For this review, take the finished solid that the model builds, in its own axes (mm). Give positions to 0.01 mm unless a question says otherwise; leave off trailing zeros. Order: outer loops, then holes, each group sorted by start corner. A loop starts at its lowest first (then second) coordinate and runs counter-clockwise, first axis right, second up. Notation, with made-up numbers: (-38, 62) - (-22, 62) arc R11 cw to (-22, 76) - close; hole circle Ø4 at (-23.75, 40.25). An arc over 180 degrees is marked (long way). One line per item, written item: value.
```python
from build123d import *

# Parameters (mm, degrees)
BOSS_EXTRUDE1_DEPTH = 5.461
BOSS_EXTRUDE2_DEPTH = 5.461
SKETCH3_W           = 5.461
SKETCH3_H           = 25.4
SKETCH3_W_2         = 19.05
SKETCH3_H_2         = 5.461
CUT_EXTRUDE1_DEPTH  = 6.461
SKETCH4_W           = 25.4
SKETCH4_H           = 10.8204
CUT_EXTRUDE2_DEPTH  = 6.461


with BuildPart() as part:
    # Sketch1 → Boss-Extrude1 (new body)
    with BuildSketch(Plane(origin=(0, 0, 0), x_dir=(1, 0, 0), z_dir=(0, 1, 0))):
        Polygon((-42.3, 45.461), (-99.45, 35.936), (-99.45, -45.979), (60.57, -45.979), (60.57, 45.461), align=None)
        with BuildLine():
            ThreePointArc((-55, 32.5), (-52.803300859, 37.803300859), (-47.5, 40))
            Line((-47.5, 40), (47.5, 40))
            ThreePointArc((47.5, 40), (52.803300859, 37.803300859), (55, 32.5))
            Line((55, 32.5), (55, -32.5))
            ThreePointArc((55, -32.5), (52.803300859, -37.803300859), (47.5, -40))
            Line((47.5, -40), (-47.5, -40))
            ThreePointArc((-47.5, -40), (-52.803300859, -37.803300859), (-55, -32.5))
            Line((-55, -32.5), (-55, 32.5))
        make_face(mode=Mode.SUBTRACT)
    extrude(amount=BOSS_EXTRUDE1_DEPTH)

    # Sketch2 → Boss-Extrude2 (add)
    with BuildSketch(Plane(origin=(0, 5.461, 0), x_dir=(1, 0, 0), z_dir=(0, 1, 0))):
        with BuildLine():
            Line((-47.5, -40), (47.5, -40))
            ThreePointArc((47.5, -40), (52.803300859, -37.803300859), (55, -32.5))
            Line((55, -32.5), (55, 32.5))
            ThreePointArc((55, 32.5), (52.803300859, 37.803300859), (47.5, 40))
            Line((47.5, 40), (-47.5, 40))
            ThreePointArc((-47.5, 40), (-52.803300859, 37.803300859), (-55, 32.5))
            Line((-55, 32.5), (-55, -32.5))
            ThreePointArc((-55, -32.5), (-52.803300859, -37.803300859), (-47.5, -40))
        make_face()
    extrude(amount=-BOSS_EXTRUDE2_DEPTH)

    # Sketch3 → Cut-Extrude1 (cut, through all)
    with BuildSketch(Plane.XZ):
        Polygon((-70.637433485, -40.738094419), (-89.428237734, -37.606293711), (-88.530454864, -32.219596493), (-69.739650615, -35.351397201), align=None)
        with Locations((-96.7195, 5.0215)):
            Rectangle(SKETCH3_W, SKETCH3_H)
        with Locations((-77.225, 43.2485)):
            Rectangle(SKETCH3_W_2, SKETCH3_H_2)
    extrude(amount=-CUT_EXTRUDE1_DEPTH, mode=Mode.SUBTRACT)

    # Sketch4 → Cut-Extrude2 (cut, through all)
    with BuildSketch(Plane(origin=(0, 5.461, 0), x_dir=(1, 0, 0), z_dir=(0, 1, 0))):
        with Locations((-6.35, -20.6375)):
            Rectangle(SKETCH4_W, SKETCH4_H)
        with Locations((-6.35, 20.6375)):
            Rectangle(SKETCH4_W, SKETCH4_H)
    extrude(amount=-CUT_EXTRUDE2_DEPTH, mode=Mode.SUBTRACT)


solid = part.part
```
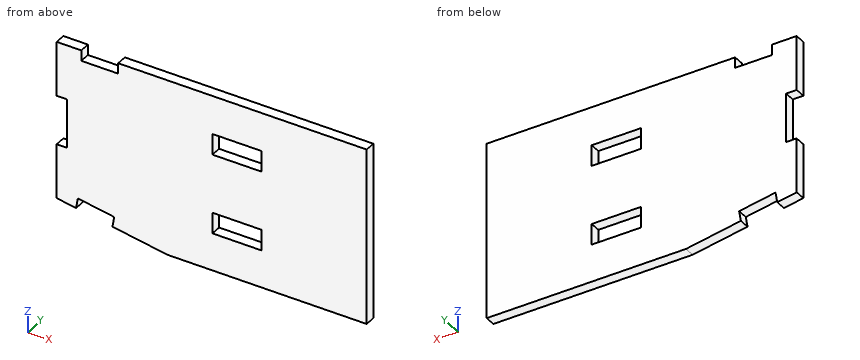
(1) Take a section at B-B (y = 2.15). Write out the cut boundary in (x, z), then the cut area to 3 significant figures.
Answers below:
outline: (-99.45, -35.94) - (-89.43, -37.61) - (-88.53, -32.22) - (-69.74, -35.35) - (-70.64, -40.74) - (-42.3, -45.46) - (60.57, -45.46) - (60.57, 45.98) - (-67.7, 45.98) - (-67.7, 40.52) - (-86.75, 40.52) - (-86.75, 45.98) - (-99.45, 45.98) - (-99.45, 17.72) - (-93.99, 17.72) - (-93.99, -7.68) - (-99.45, -7.68) - close; hole (-19.05, -26.05) - (6.35, -26.05) - (6.35, -15.23) - (-19.05, -15.23) - close; hole (-19.05, 15.23) - (6.35, 15.23) - (6.35, 26.05) - (-19.05, 26.05) - close
area: 13,500 mm^2
(2) For P1, Ø2.5, axis at x = -95.5, y = 3, coming from the -Z side, flat-tipped, find the tip position at first contact; note if it passes through.
Answers below:
P1: stops at z = -36.8
(3) Take a section at D-D (x = -64). Write out the cut boundary in (y, z).
Answers below:
outline: (0, -41.84) - (5.46, -41.84) - (5.46, 45.98) - (0, 45.98) - close
(4) Wall thickness on line 1 (Z direction, x = -3, y = 3.45); line 2 (X direction, y = 2.4, z = -19); line 3 (X direction, y = 4.7, z = 10): over which ranges is each line inside the solid? List them lowest first. Write a range as from..to.
Answers below:
line 1: z = -45.46..-26.05, -15.23..15.23, 26.05..45.98
line 2: x = -99.45..-19.05, 6.35..60.57
line 3: x = -93.99..60.57
(5) Take a section at C-C (z = -6). Write out the cut boundary in (x, y), then the cut area to 3 significant figures.
Answers below:
outline: (-93.99, 0) - (60.57, 0) - (60.57, 5.46) - (-93.99, 5.46) - close
area: 844 mm^2
(6) Take a section at A-A (x = -9.5). Write out the cut boundary in (y, z), then the cut area to 3 significant figures.
Answers below:
outline: (0, -45.46) - (5.46, -45.46) - (5.46, -26.05) - (0, -26.05) - close; (0, -15.23) - (5.46, -15.23) - (5.46, 15.23) - (0, 15.23) - close; (0, 26.05) - (5.46, 26.05) - (5.46, 45.98) - (0, 45.98) - close
area: 381 mm^2
